Verification items for the finished model (mm, model axes). A direction names the side the tool comes from. Round coordinates to 2 decimals unless told otherwise and drop trailing zeros. Order: outer loops, then holes, each group sorted by start corner. A loop starts at its lowest first (then second) coordinate and runs counter-clockwise, first axis right, second up. Notation, with made-up numbers: M -26,17.25 L -8,17.25 A19 cw -8,28.25 Z; hole C 34.25,83 d1. An arc over 180 degrees is marked long. Use one line per item in the form item = value. Start each with the question number.
Item 1: Cross-section at D-D on x = 138. Enter the section's corners in (y, z).
Item 2: Release check for a two-part mould opening along X. For faces 3 (the flat face through (70.845, 34.915, -3.131)), 4 (the flat face through (73.062, -28.565, -3.131)), 5 (the flat face through (71, -27, -6.35)), 6 (the cylindrical face through (49.695, 1.453, -3.131)) record: +X half, -X half, draft (parallel to the pull), parting line (faces both ways), or undercut.
Item 3: Thickness scan on probe 1 along Y at (x, z) = (102, -1.5); probe 2 along X at (y, z) = (24.5, -5.75); probe 3 along Y at (x, z) = (67.5, -6). Record the ranges inside material, lowest first. Write a range as [from, to].
Item 4: Cross-section at B-B on z = -4.75. Enter the section's corners in (x, y), then the cut area to 3 significant figures.
Item 5: Cross-section at A-A on y = 2. Enter the section's corners in (x, z), then the cut area to 3 significant figures.
Item 6: Tool access check on faces 1 (the flat face through (71, -27, 0)), 2 (the flat face through (73.934, -22.152, -3.131)). Record the directions out of +Z, -Z, +X, -X, +Y, -Y that give a thin tool (end or side, any length) a straight path to the whole face; none if there is none.
Item 7: Cross-section at C-C on y = -7. Enter the section's corners in (x, z), then the cut area to 3 significant figures.
Item 8: Go/stop test with flat-tipped pins: pin 1 Ø1 at (y, z) = (8.5, -5.5) entering from -X; pin 2 Ø3 at (y, z) = (-10.5, -1) entering from -X; pin 3 Ø1.5 at (x, y) = (29, 4.5) entering from +Z; pin 4 Ø1 at (y, z) = (-12.5, -1) entering from +X. Record where each tip stops, or that it passes through.
Autodesk Inventor part; units mm, degrees
ref_plane "YZ Plane" through (0, 0, 0) normal (1, 0, 0) x (0, 1, 0)
ref_plane "XZ Plane" through (0, 0, 0) normal (0, 1, 0) x (-1, 0, 0)
ref_plane "XY Plane" through (0, 0, 0) normal (0, 0, 1) x (1, 0, 0)
sketch "Sketch1" plane through (0, 0, 0) normal (0, 0, 1) x (1, 0, 0)
  circle A0 centre (17.9784, 0) radius 31.75
  circle A1 centre (125.9284, 6.35) radius 31.75
  line L0 (124.0639, 38.0452) -> (16.1139, 31.6952)
  line L1 (19.8428, -31.6952) -> (127.7928, -25.3452)
  line L2 (35.504, 26.4748) -> (105.4197, 30.5875)
  line L3 (108.4028, -20.1248) -> (38.487, -24.2375)
  line L4 (35.504, 26.4748) -> (16.1139, 31.6952)
  line L5 (38.487, -24.2375) -> (17.9784, -31.75)
  line L6 (108.4028, -20.1248) -> (127.7928, -25.3452)
  line L7 (105.4197, 30.5875) -> (124.0639, 38.0452)
  point P0 (0, 0)
  dimension "d0" = 107.95
  dimension "d1" = 6.35
  dimension "d2" = 63.5
  dimension "d3" = 63.5
  dimension "d4" = 6.35
  dimension "d5" = 6.35
extrude "Extrusion1" add sketch "Sketch1" against normal blind 6.35 contours A0 L5 L4 | L4 A0 | A0 L0 A1 L2 | L3 A1 L1 A0 | A0 L5 | L7 A1 L6 | A1 L7 | L6 A1
properties part number "shooterchain"
Output values:
q1.outline = M -23.02,-6.35 L 35.72,-6.35 L 35.72,0 L -23.02,0 Z
q2.face_3 = -X half
q2.face_4 = +X half
q2.face_5 = draft
q2.face_6 = undercut
q3.probe_1 = [-26.86, -20.5], [-14.52, 27.22], [30.39, 36.75]
q3.probe_2 = [-2.22, 38.17], [99.88, 151.98]
q3.probe_3 = [-28.89, -22.53], [28.36, 34.72]
q4.outline = M 16.11,31.7 A31.75 ccw 19.84,-31.7 L 127.79,-25.35 A31.75 ccw 124.06,38.05 Z; hole M 35.5,26.47 A31.75 cw 38.49,-24.24 L 108.4,-20.12 A31.75 cw 105.42,30.59 Z
q4.area = 7,380 mm2
q5.outline = M -13.71,-6.35 L 49.67,-6.35 L 49.67,0 L -13.71,0 Z; M 94.48,-6.35 L 157.38,-6.35 L 157.38,0 L 94.48,0 Z
q5.area = 802 mm2
q6.face_1 = +Z, +X, -X, +Y, -Y
q6.face_2 = +Z, -Z
q7.outline = M -12.99,-6.35 L 48.95,-6.35 L 48.95,0 L -12.99,0 Z; M 97.12,-6.35 L 154.74,-6.35 L 154.74,0 L 97.12,0 Z
q7.area = 759 mm2
q8.pin_1 = -12.75
q8.pin_2 = -12.47
q8.pin_3 = 0
q8.pin_4 = 151.84
